Geometry: final body of the model. Coordinates: model frame, mm. A direction names the side the tool comes from. Give positions to 0.01 mm unless a question says otherwise; leave off trailing zeros. Loops run counter-clockwise (first coordinate to the right, second up) from the corner with the lowest first, then second, coordinate; pieces in that order, holes last.
from build123d import *

# Parameters (mm, degrees)
SKETCH_1_R                   = 22
EXTRUDE_1_DEPTH              = 6
SKETCH_2_R                   = 15
EXTRUDE_2_DEPTH              = 10
EXTRUDE_START                = 15
SKETCH_3_R                   = 22
SKETCH_3_R_2                 = 2
EXTRUDE_3_DEPTH              = 15
SKETCH_4_R                   = 1.5
CUT_EXTRUDE_1_DEPTH          = 40.912404087
SKETCH_5_R                   = 4.5
CUT_EXTRUDE_2_DEPTH          = 40.91240426
HOLE_WIZARD_M4_1_D           = 3.3
HOLE_WIZARD_M4_1_CSINK_D     = 4.05
HOLE_WIZARD_M4_1_CSINK_ANGLE = 90
SKETCH_8_R                   = 1.5
CUT_EXTRUDE_3_DEPTH          = 40.91240426
SKETCH_9_R                   = 4.5
CUT_EXTRUDE_4_DEPTH          = 40.91240426
HOLE_WIZARD_M4_2_D           = 3.3
HOLE_WIZARD_M4_2_CSINK_D     = 4.05
HOLE_WIZARD_M4_2_CSINK_ANGLE = 90
SKETCH_11_R                  = 4
CUT_EXTRUDE_5_DEPTH          = 15
SKETCH_12_R                  = 5
CUT_EXTRUDE_6_DEPTH          = 15
SKETCH_13_R                  = 10
CUT_EXTRUDE_7_DEPTH          = 10


with BuildPart() as part:
    # 草图1 → 凸台-拉伸1 (new, symmetric)
    with BuildSketch(Plane.XY):
        Circle(SKETCH_1_R)
    extrude(amount=EXTRUDE_1_DEPTH, both=True)

    # 草图2 → 凸台-拉伸2 (add, symmetric)
    with BuildSketch(Plane.XY):
        Circle(SKETCH_2_R)
    extrude(amount=EXTRUDE_2_DEPTH, both=True)

    # 草图3 → 凸台-拉伸3 (add)
    with BuildSketch(Plane.XY.offset(10).offset(EXTRUDE_START)):
        Circle(SKETCH_3_R)
        with Locations(Location((0, 13.75, 0), (0, 0, 144.501487602))):
            Circle(SKETCH_3_R_2, mode=Mode.SUBTRACT)
        with Locations(Location((0, -13.75, 0), (0, 0, 180))):
            Circle(SKETCH_3_R_2, mode=Mode.SUBTRACT)
    extrude_3 = extrude(amount=-EXTRUDE_3_DEPTH)

    # 草图4 → 切除-拉伸1 (cut, through all)
    with BuildSketch(Plane(origin=(0, 0, 0), x_dir=(1, 0, 0), z_dir=(0, 1, 0))):
        with Locations(Location((-16, -20, 0), (0, 0, 270))):
            Circle(SKETCH_4_R)
    extrude(amount=-CUT_EXTRUDE_1_DEPTH, mode=Mode.SUBTRACT)

    # 草图5 → 切除-拉伸2 (cut, through all)
    with BuildSketch(Plane(origin=(0, 0, 0), x_dir=(1, 0, 0), z_dir=(0, 1, 0))):
        with Locations(Location((-16, -20, 0), (0, 0, 90))):
            Circle(SKETCH_5_R)
    extrude(amount=CUT_EXTRUDE_2_DEPTH, mode=Mode.SUBTRACT)

    # M4 螺纹孔1 (through all)
    with Locations(Plane(origin=(0, 0, 0), x_dir=(1, 0, 0), z_dir=(0, 1, 0))):
        with Locations((-16, -20)):
            CounterSinkHole(HOLE_WIZARD_M4_1_D / 2, HOLE_WIZARD_M4_1_CSINK_D / 2, counter_sink_angle=HOLE_WIZARD_M4_1_CSINK_ANGLE)

    # 镜向1: 凸台-拉伸3 across plane
    add(extrude_3.mirror(Plane.XY))

    # 草图8 → 切除-拉伸3 (cut, through all)
    with BuildSketch(Plane(origin=(0, 0, 0), x_dir=(1, 0, 0), z_dir=(0, 1, 0))):
        with Locations(Location((-16, 20, 0), (0, 0, 90))):
            Circle(SKETCH_8_R)
    extrude(amount=CUT_EXTRUDE_3_DEPTH, mode=Mode.SUBTRACT)

    # 草图9 → 切除-拉伸4 (cut, through all)
    with BuildSketch(Plane(origin=(0, 0, 0), x_dir=(1, 0, 0), z_dir=(0, 1, 0))):
        with Locations(Location((-16, 20, 0), (0, 0, 270))):
            Circle(SKETCH_9_R)
    extrude(amount=-CUT_EXTRUDE_4_DEPTH, mode=Mode.SUBTRACT)

    # M4 螺纹孔2 (through all)
    with Locations(Plane(origin=(-16, 0, -20), x_dir=(0, 0, -1), z_dir=(0, -1, 0))):
        with Locations((0, 0)):
            CounterSinkHole(HOLE_WIZARD_M4_2_D / 2, HOLE_WIZARD_M4_2_CSINK_D / 2, counter_sink_angle=HOLE_WIZARD_M4_2_CSINK_ANGLE)

    # 草图11 → 切除-拉伸5 (cut)
    with BuildSketch(Plane.XY.offset(25)):
        Circle(SKETCH_11_R)
    extrude(amount=-CUT_EXTRUDE_5_DEPTH, mode=Mode.SUBTRACT)

    # 草图12 → 切除-拉伸6 (cut)
    with BuildSketch(Plane(origin=(0, 0, -25), x_dir=(-1, 0, 0), z_dir=(0, 0, -1))):
        Circle(SKETCH_12_R)
    extrude(amount=-CUT_EXTRUDE_6_DEPTH, mode=Mode.SUBTRACT)

    # 草图13 → 切除-拉伸7 (cut, symmetric)
    with BuildSketch(Plane.XY):
        Circle(SKETCH_13_R)
    extrude(amount=CUT_EXTRUDE_7_DEPTH, both=True, mode=Mode.SUBTRACT)


solid = part.part
Item 1: Section query B-B on y = -2. Give the number of separate pieces and of enclosed holes in the cut face, plus the area to 3 significant figures.
Values follow:
separate pieces: 2
enclosed holes: 2
area: 1,370 mm2
Item 2: Set-up query: faces 1 (the face through (0.26, -15.733, 17.605)), 2 (the face through (-0.867, -3.905, 17.605)), 3 (the face through (-14.35, -8.64, 19.93)), 4 (the face through (0.415, 11.794, -17.605)), 5 (the face through (-14.985, 0.66, -7.972)). Return all of +Z, -Z, +X, -X, +Y, -Y with unobstructed straight access to the full face (end or side cutting, diameter ignored); none if empty.
Values follow:
face 1: +Z
face 2: +Z, -Z
face 3: +Y, -Y
face 4: -Z
face 5: none
Item 3: Section query A-A on z = 20. Return loops of the section in (x, y) (3 decimals), plus the area to 3 significant figures.
Values follow:
outline: (-20.5, 0) - (-20.5, 7.984) arc R22 ccw to (-17.65, -13.133) - (-17.65, -0.375) - (-18.025, 0) - close; (-14.35, -16.676) arc R22 ccw (long way) to (-11.5, 18.755) - (-11.5, 0) - (-13.975, 0) - (-14.35, -0.375) - close; hole circle Ø8 at (0, 0); hole circle Ø4 at (0, -13.75); hole circle Ø4 at (0, 13.75)
area: 1,260 mm2
Item 4: Draft query along Y for faces 6 (the face through (20.984, 6.608, -17.605)), 7 (the face through (0, -5, 25)), 8 (the face through (-5, -2, -10)). Return one class per face: +Y half, -Y half, draft (parallel to the pull), parting line (faces both ways), or undercut.
Values follow:
face 6: parting line
face 7: draft
face 8: undercut
Item 5: Ray query, probe 1 along Z at (x, y) = (1, 16); probe 2 along Z at (x, y) = (-16, -13.5); probe 3 along X at (y, z) = (-3.5, -17). Return the intervals inside material, ascending.
Values follow:
probe 1: z = -25 to -10, -6 to 6, 10 to 25
probe 2: z = -25 to -24.5, -15.5 to -10, -6 to 6, 10 to 18.35, 21.65 to 25
probe 3: x = -21.72 to -19.35, -12.65 to -3.57, 3.57 to 21.72
Item 6: Pin query (flat end, axial travel): pin 1 (10 mm diameter, centred on x = -16.5, z = -19.5, fed in from -Y) (3 decimals); pin 2 (3 mm diameter, centred on x = 0, y = 13.75, fed in from -Z); pin 3 (5.5 mm diameter, centred on x = -16, z = 20, fed in from -Y). Return the tip coordinate at first contact, or that it passes through.
Values follow:
pin 1: stops at y = -18.755
pin 2: stops at z = -10
pin 3: stops at y = -17.56
